The model under review builds one solid part; all positions refer to its coordinate system, in mm. Face numbers are marked on the shaded views. A direction names the side the tool comes from. Round coordinates to 2 decimals unless told otherwise and drop trailing zeros. Order: outer loops, then holes, each group sorted by start corner. A loop starts at its lowest first (then second) coordinate and runs counter-clockwise, first axis right, second up.
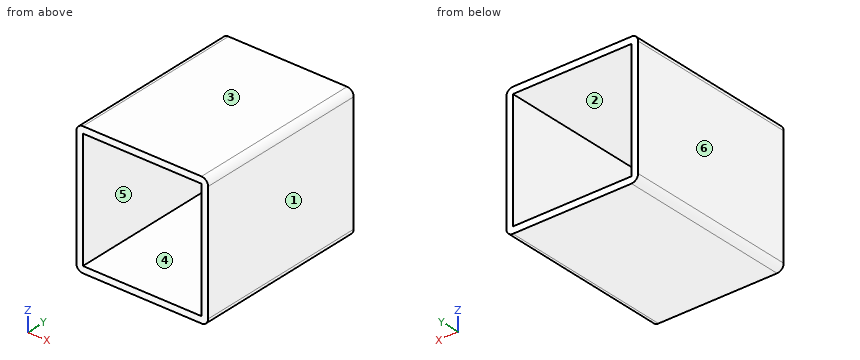
```python
from build123d import *

# Parameters (mm, degrees)
SKETCH1_W           = 60
SKETCH1_H           = 60
SKETCH1_W_2         = 54
SKETCH1_H_2         = 54
BOSS_EXTRUDE1_DEPTH = 80
FILLET2_R           = 3


with BuildPart() as part:
    # Sketch1 → Boss-Extrude1 (new body)
    with BuildSketch(Plane(origin=(0, 0, 0), x_dir=(1, 0, 0), z_dir=(0, 1, 0))):
        with Locations((30, 30)):
            Rectangle(SKETCH1_W, SKETCH1_H)
        with Locations((30, 30)):
            Rectangle(SKETCH1_W_2, SKETCH1_H_2, mode=Mode.SUBTRACT)
    extrude(amount=BOSS_EXTRUDE1_DEPTH)

    # Fillet2
    fillet2_edges = [part.edges().sort_by_distance(p)[0] for p in [
        (0, 40, -60),
        (60, 40, -60),
        (60, 40, 0),
        (0, 40, 0),
    ]]
    fillet(fillet2_edges, radius=FILLET2_R)


solid = part.part
```
(1) Draft analysis for pull direction Z (two halves, no side actions). For the marked faces 3, 4, 5 and 6, state which applies: pulls with the +Z half, pulls with the -Z half, needs draft (parallel to the pull), parting line crosses it, or undercut.
Data:
face 3: pulls with the +Z half
face 4: undercut
face 5: undercut
face 6: needs draft
(2) Insertion check: pin 1 (8 mm diameter, centred on x = 44.5, z = -49.5, fed in from -Y) (3 decimals). The pin has a flat end and moves straight along its axis. Give the tip position at first contact, or say it passes through.
Data:
pin 1: passes through
(3) Consider section A-A (z = -20.5). Write out the cut boundary in (x, y).
Data:
outline: (0, 0) - (3, 0) - (3, 80) - (0, 80) - close; (57, 0) - (60, 0) - (60, 80) - (57, 80) - close
(4) Consider section B-B (x = 26.5). Write out the cut boundary in (y, z).
Data:
outline: (0, -60) - (80, -60) - (80, -57) - (0, -57) - close; (0, -3) - (80, -3) - (80, 0) - (0, 0) - close
(5) For the marked faces 1 and 2, list the 3-axis set-ups (+Z, -Z, +X, -X, +Y, -Y) from which the entire face can be reached by the end or side of a thin tool; tool diameter is ignored.
Data:
face 1: +Z, -Z, +X, +Y, -Y
face 2: +Y, -Y
(6) To check wall thickness, follow probe 1 along X at (y, z) = (60, -36); probe 2 along Z at (x, y) = (41, 59.5). State the ranges of each line that lie inside material, in increasing order.
Data:
probe 1: x = 0 to 3, 57 to 60
probe 2: z = -60 to -57, -3 to 0
(7) Consider section C-C (y = 24.5). Write out the cut boundary in (x, z), and give its area (3 significant figures).
Data:
outline: (0, -57) arc R3 ccw to (3, -60) - (57, -60) arc R3 ccw to (60, -57) - (60, -3) arc R3 ccw to (57, 0) - (3, 0) arc R3 ccw to (0, -3) - close; hole (3, -57) - (57, -57) - (57, -3) - (3, -3) - close
area: 676 mm2
